```python
from build123d import *

# Parameters (mm, degrees)
EXTRUDE_1_DEPTH     = 3
SKETCH_2_W          = 40
SKETCH_2_H          = 3
EXTRUDE_2_DEPTH     = 40
SKETCH_3_R          = 2.5
CUT_EXTRUDE_1_DEPTH = 1.5
SKETCH_4_R          = 1.5
CUT_EXTRUDE_2_DEPTH = 66.812232905
SKETCH_5_R          = 1.5
CUT_EXTRUDE_3_DEPTH = 67.76825593
FILLET_1_R          = 3
CUT_EXTRUDE_4_REACH = 68.768


with BuildPart() as part:
    # 草图1 → 凸台-拉伸1 (new body)
    with BuildSketch(Plane.XY):
        with BuildLine():
            Line((-20, 0), (20, 0))
            Line((20, 0), (20, 27))
            ThreePointArc((20, 27), (0, 47), (-20, 27))
            Line((-20, 27), (-20, 0))
        make_face()
    extrude(amount=EXTRUDE_1_DEPTH)

    # 草图2 → 凸台-拉伸2 (add)
    with BuildSketch(Plane.XY.offset(3)):
        with Locations((0, 1.5)):
            Rectangle(SKETCH_2_W, SKETCH_2_H)
    extrude(amount=EXTRUDE_2_DEPTH)

    # 草图3 → 切除-拉伸1 (cut)
    with BuildSketch(Plane(origin=(0, 0, 0), x_dir=(-1, 0, 0), z_dir=(0, 0, -1))):
        with Locations((-15.5, 27)):
            Circle(SKETCH_3_R)
        with Locations((-7.75, 40.423393759)):
            Circle(SKETCH_3_R)
        with Locations((7.75, 40.423393759)):
            Circle(SKETCH_3_R)
        with Locations((15.5, 27)):
            Circle(SKETCH_3_R)
        with Locations((7.75, 13.576606241)):
            Circle(SKETCH_3_R)
        with Locations((-7.75, 13.576606241)):
            Circle(SKETCH_3_R)
    extrude(amount=-CUT_EXTRUDE_1_DEPTH, mode=Mode.SUBTRACT)

    # 草图4 → 切除-拉伸2 (cut, through all)
    with BuildSketch(Plane(origin=(0, 0, 1.5), x_dir=(-1, 0, 0), z_dir=(0, 0, -1))):
        with Locations((-15.5, 27)):
            Circle(SKETCH_4_R)
        with Locations((-7.75, 40.423393759)):
            Circle(SKETCH_4_R)
        with Locations((7.75, 40.423393759)):
            Circle(SKETCH_4_R)
        with Locations((15.5, 27)):
            Circle(SKETCH_4_R)
        with Locations((7.75, 13.576606241)):
            Circle(SKETCH_4_R)
        with Locations((-7.75, 13.576606241)):
            Circle(SKETCH_4_R)
    extrude(amount=-CUT_EXTRUDE_2_DEPTH, mode=Mode.SUBTRACT)

    # 草图5 → 切除-拉伸3 (cut, through all)
    with BuildSketch(Plane.XZ):
        with Locations(Location((-15, 35, 0), (0, 0, 270))):
            Circle(SKETCH_5_R)
        with Locations(Location((15, 35, 0), (0, 0, 270))):
            Circle(SKETCH_5_R)
        with Locations(Location((-14.39414679, 11, 0), (0, 0, 270))):
            Circle(SKETCH_5_R)
        with Locations(Location((15, 11, 0), (0, 0, 270))):
            Circle(SKETCH_5_R)
    extrude(amount=-CUT_EXTRUDE_3_DEPTH, mode=Mode.SUBTRACT)

    # 圆角1
    fillet_1_edges = [part.edges().sort_by_distance(p)[0] for p in [
        (20, 1.5, 43),
        (-20, 1.5, 43),
    ]]
    fillet(fillet_1_edges, radius=FILLET_1_R)

    # 草图6 → 切除-拉伸4 (cut, up to next)
    with BuildSketch(Plane(origin=(0, 0, 0), x_dir=(-1, 0, 0), z_dir=(0, 0, -1)), mode=Mode.PRIVATE) as cut_extrude_4_sk1:
        with BuildLine():
            Line((-6.5, 34), (-6.5, 20))
            ThreePointArc((-6.5, 20), (0, 13.5), (6.5, 20))
            Line((6.5, 20), (6.5, 34))
            ThreePointArc((6.5, 34), (0, 40.5), (-6.5, 34))
        make_face()
    cut_extrude_4_tool1 = extrude(cut_extrude_4_sk1.sketch, amount=-CUT_EXTRUDE_4_REACH, mode=Mode.PRIVATE) & part.part
    add(cut_extrude_4_tool1.solids().sort_by_distance((0, 27, 0))[0], mode=Mode.SUBTRACT)


solid = part.part
```
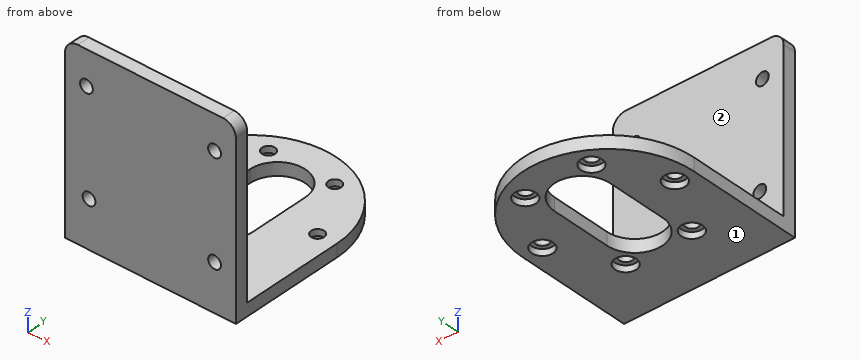
Geometry check sheet. Reference: the model listing, model coordinates, mm. Face numbers are marked on the shaded views. A direction names the side the tool comes from. Round coordinates to 2 decimals unless told otherwise and drop trailing zeros. Order: outer loops, then holes, each group sorted by start corner. A loop starts at its lowest first (then second) coordinate and runs counter-clockwise, first axis right, second up. Notation, with made-up numbers: (43, 78.25) - (99, 78.25) arc R21 cw to (99, 83.25) - close; hole circle Ø2 at (-17, 18.25). An arc over 180 degrees is marked (long way). Use a Markdown table: item, result. Add a question column.
1) Thickness scan on line 1 along X through (y, z) = (2.1, 35); line 2 along Z through (x, y) = (-17.5, 21). Record the ranges inside material, lowest first.
2) Section check B-B (x = 0). Record the cut outline in (y, z).
3) Gauge pin test, flat ends, axial feed: P1, Ø5, axis at x = -15, z = 38.5, coming from the +Y side; P2, Ø6.5, axis at x = -7.75, y = 13.58, coming from the +Z side; P3, Ø2.5, axis at x = 7.5, y = 41.5, coming from the -Z side; P4, Ø2.5, axis at x = 15.5, y = 27, coming from the -Z side. Record the tip position at first contact, or that the pin passes through.
4) Section check A-A (z = 11). Record the cut outline in (x, y).
5) Section check C-C (x = -7.75). Record the cut outline in (y, z).
6) Set-up check for the marked faces 1 and 2: record each of +Z, -Z, +X, -X, +Y, -Y from which the full face is reachable in a straight line by a thin tool's end or side.
7) Section check D-D (y = 19). Record the cut outline in (x, z), then the cut area to 3 significant figures.
Established:
| question | item | result |
|---|---|---|
| 1 | line 1 | -20 to -16.5, -13.5 to 13.5, 16.5 to 20 |
| 1 | line 2 | 0 to 3 |
| 2 | outline | (0, 0) - (13.5, 0) - (13.5, 3) - (3, 3) - (3, 43) - (0, 43) - close; (40.5, 0) - (47, 0) - (47, 3) - (40.5, 3) - close |
| 3 | P1 | y = 3 |
| 3 | P2 | z = 3 |
| 3 | P3 | z = 1.5 |
| 3 | P4 | through |
| 4 | outline | (-20, 0) - (-15.89, 0) - (-15.89, 3) - (-20, 3) - close; (-12.89, 0) - (13.5, 0) - (13.5, 3) - (-12.89, 3) - close; (16.5, 0) - (20, 0) - (20, 3) - (16.5, 3) - close |
| 5 | outline | (0, 0) - (11.08, 0) - (11.08, 1.5) - (12.08, 1.5) - (12.08, 3) - (3, 3) - (3, 43) - (0, 43) - close; (15.08, 1.5) - (16.08, 1.5) - (16.08, 0) - (37.92, 0) - (37.92, 1.5) - (38.92, 1.5) - (38.92, 3) - (15.08, 3) - close; (41.92, 1.5) - (42.92, 1.5) - (42.92, 0) - (45.44, 0) - (45.44, 3) - (41.92, 3) - close |
| 6 | face 1 | -Z, +X, -X, +Y, -Y |
| 6 | face 2 | +Z, +X, -X, +Y |
| 7 | outline | (-20, 0) - (-6.42, 0) - (-6.42, 3) - (-20, 3) - close; (6.42, 0) - (20, 0) - (20, 3) - (6.42, 3) - close |
| 7 | area | 81.5 mm2 |
